Design review of the part built by this model. Coordinates are the model's own, in mm. A direction names the side the tool comes from. Coordinates: 2 decimals unless noted, no trailing zeros. Order: outer loops, then holes, each group sorted by start corner. A loop starts at its lowest first (then second) coordinate and runs counter-clockwise, first axis right, second up. Notation, with made-up numbers: M 51,-16 L 109,-16 A30 cw 109,11 Z; hole C 10.25,-39 d7. An arc over 180 degrees is marked long. Answer as a JSON object with one key per item and string values.
from build123d import *

# Parameters (mm, degrees)
SKETCH1_W           = 75
SKETCH1_H           = 53
SKETCH1_R           = 1.75
BOSS_EXTRUDE8_DEPTH = 6
SKETCH8_R           = 1.6
CUT_EXTRUDE1_DEPTH  = 10
CUT_EXTRUDE2_START  = -43
SKETCH8_3_R         = 1.6
CUT_EXTRUDE2_DEPTH  = 10


with BuildPart() as part:
    # Sketch1 → Boss-Extrude8 (new body)
    with BuildSketch(Plane(origin=(0, 0, 0), x_dir=(1, 0, 0), z_dir=(0, 1, 0))):
        with Locations((37.5, -26.5)):
            Rectangle(SKETCH1_W, SKETCH1_H)
        with Locations(Location((71.25, -6.5, 0), (0, 0, 270))):
            Circle(SKETCH1_R, mode=Mode.SUBTRACT)
        with Locations(Location((3.75, -6.5, 0), (0, 0, 270))):
            Circle(SKETCH1_R, mode=Mode.SUBTRACT)
        with Locations(Location((71.25, -46.5, 0), (0, 0, 270))):
            Circle(SKETCH1_R, mode=Mode.SUBTRACT)
        with Locations(Location((3.75, -46.5, 0), (0, 0, 270))):
            Circle(SKETCH1_R, mode=Mode.SUBTRACT)
    extrude(amount=BOSS_EXTRUDE8_DEPTH)

    # Sketch8 → Cut-Extrude1 (cut)
    with BuildSketch(Plane.XY.offset(53)):
        with Locations((17.5, 3)):
            Circle(SKETCH8_R)
        with Locations((57.5, 3)):
            Circle(SKETCH8_R)
    extrude(amount=-CUT_EXTRUDE1_DEPTH, mode=Mode.SUBTRACT)

    # Sketch8<3> → Cut-Extrude2 (cut)
    with BuildSketch(Plane.XY.offset(53).offset(CUT_EXTRUDE2_START)):
        with Locations((17.5, 3)):
            Circle(SKETCH8_3_R)
        with Locations((57.5, 3)):
            Circle(SKETCH8_3_R)
    extrude(amount=-CUT_EXTRUDE2_DEPTH, mode=Mode.SUBTRACT)


solid = part.part
1) Add section C-C (y = 3). State the section outline as (x, z) points, and give its area (3 significant figures).
Taken from the geometry:
{"outline": "M 0,0 L 15.9,0 L 15.9,10 L 19.1,10 L 19.1,0 L 55.9,0 L 55.9,10 L 59.1,10 L 59.1,0 L 75,0 L 75,53 L 59.1,53 L 59.1,43 L 55.9,43 L 55.9,53 L 19.1,53 L 19.1,43 L 15.9,43 L 15.9,53 L 0,53 Z; hole C 3.75,6.5 d3.5; hole C 3.75,46.5 d3.5; hole C 71.25,6.5 d3.5; hole C 71.25,46.5 d3.5", "area": "3,810 mm2"}
2) To check wall thickness, follow L1, parallel to Z at x = 71.25, y = 1.9; L2, parallel to X at y = 2.8, z = 6.5; L3, parallel to X at y = 1, z = 8. State the ranges of each line that lie inside material, in increasing order.
Taken from the geometry:
{"L1": "z = 0 to 4.75, 8.25 to 44.75, 48.25 to 53", "L2": "x = 0 to 2, 5.5 to 15.91, 19.09 to 55.91, 59.09 to 69.5, 73 to 75", "L3": "x = 0 to 2.85, 4.65 to 70.35, 72.15 to 75"}
3) Tool access review of faces 1 (the cylindrical face through (69.54, 2.96, 6.12)), 2 (the cylindrical face through (58.98, 2.39, 48.07)), 3 (the flat face through (57, 3, 10)): name each direction out of +Z, -Z, +X, -X, +Y, -Y from which nothing blocks a thin tool from reaching the whole face with its end or side.
Taken from the geometry:
{"face 1": "+Y, -Y", "face 2": "+Z", "face 3": "-Z"}
4) Add section A-A (z = 46.5). State the section outline as (x, y) points.
Taken from the geometry:
{"outline": "M 0,0 L 2,0 L 2,6 L 0,6 Z; M 5.5,0 L 69.5,0 L 69.5,6 L 5.5,6 Z; M 73,0 L 75,0 L 75,6 L 73,6 Z; hole C 17.5,3 d3.2; hole C 57.5,3 d3.2"}
5) Add section D-D (x = 17.5). State the section outline as (y, z) points.
Taken from the geometry:
{"outline": "M 0,0 L 1.4,0 L 1.4,10 L 4.6,10 L 4.6,0 L 6,0 L 6,53 L 4.6,53 L 4.6,43 L 1.4,43 L 1.4,53 L 0,53 Z"}
6) Insertion check: pin 1 Ø5.5 at (x, z) = (3.75, 46.5) entering from -Y; pin 2 Ø3 at (x, y) = (57.5, 3) entering from +Z; pin 3 Ø1.6 at (x, y) = (57, 3.5) entering from -Z; pin 4 Ø3 at (x, z) = (3.75, 6.5) entering from +Y. Each pin has a flat end and moves straight along its axis. Give the tip position at first contact, or say it passes through.
Taken from the geometry:
{"pin 1": "stops at y = 0", "pin 2": "stops at z = 43", "pin 3": "stops at z = 10", "pin 4": "passes through"}
7) Mouldability with a two-part tool opening along Z and no side actions: class faces 4 (the flat face through (17, 3, 43)), 5 (the cylindrical face through (70.58, 2.958, 48.117)), 6 (the cylindrical face through (15.9, 3.07, 48.07)) as released by +Z, released by -Z, zero draft, split by the parting line, or undercut.
Taken from the geometry:
{"face 4": "released by +Z", "face 5": "undercut", "face 6": "zero draft"}
8) Add section B-B (x = 3.75). State the section outline as (y, z) points.
Taken from the geometry:
{"outline": "M 0,0 L 6,0 L 6,4.75 L 0,4.75 Z; M 0,8.25 L 6,8.25 L 6,44.75 L 0,44.75 Z; M 0,48.25 L 6,48.25 L 6,53 L 0,53 Z"}
